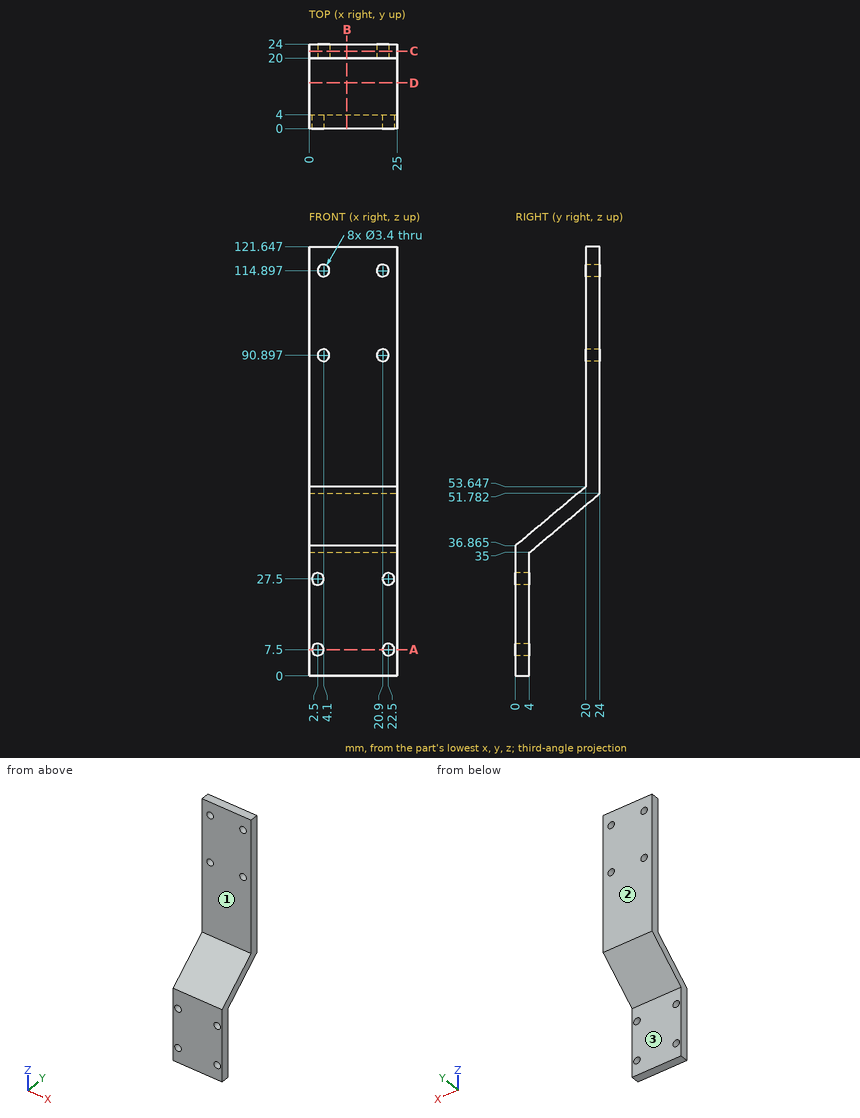
Verification items for this drawing (mm, ordinates from the low corner). A direction names the side the tool comes from. Give positions to 0.01 mm unless a question says otherwise; leave off trailing zeros. Loops run counter-clockwise (first coordinate to the right, second up) from the corner with the lowest first, then second, coordinate; pieces in that order, holes last. Notation, with made-up numbers: M -9,36.25 L 12,36.25 A16 cw 12,53.25 Z; hole C -25.5,18 d11. An arc over 180 degrees is marked long. Return JSON: item names as keys, results as strings. Group by question number.
1. Cross-section at B-B on x = 10.75. Record the boundary of the cut face in (y, z) (1 decimal), plus the area to 3 significant figures.
2. Cross-section at C-C on y = 22. Record the boundary of the cut face in (x, z), plus the area to 3 significant figures.
3. Cross-section at D-D on y = 13. Record the boundary of the cut face in (x, z), plus the area to 3 significant figures.
4. Tool access check on the marked faces 1, 2 and 3. Record the directions out of +Z, -Z, +X, -X, +Y, -Y that give a thin tool (end or side, any length) a straight path to the whole face; none if there is none.
5. Thickness scan on L1, parallel to X at y = 1.6, z = 7.5; L2, parallel to Z at x = 20.9, y = 22.6; L3, parallel to Z at x = 22.5, y = 2. Record the ranges inside material, lowest first.
6. Go/stop test with flat-tipped pins: pin 1 (10 mm diameter, centred on x = 20.5, y = 13.5, fed in from -Z); pin 2 (12 mm diameter, centred on x = 10.5, z = 80.5, fed in from -Y); pin 3 (4.5 mm diameter, centred on x = 4.1, z = 90.9, fed in from +Y); pin 4 (4 mm diameter, centred on x = 2.5, z = 7.5, fed in from +Y). Record where each tip stops, or that it passes through.
7. Cross-section at A-A on z = 7.5. Record the boundary of the cut face in (x, y).
Return value:
{
 "1": {"outline": "M 0,0 L 4,0 L 4,35 L 24,51.8 L 24,121.6 L 20,121.6 L 20,53.6 L 0,36.9 Z", "area": "524 mm^2"},
 "2": {"outline": "M 0,50.1 L 25,50.1 L 25,121.65 L 0,121.65 Z; hole C 4.1,90.9 d3.4; hole C 4.1,114.9 d3.4; hole C 20.9,90.9 d3.4; hole C 20.9,114.9 d3.4", "area": "1,750 mm^2"},
 "3": {"outline": "M 0,42.55 L 25,42.55 L 25,47.77 L 0,47.77 Z", "area": "131 mm^2"},
 "4": {"face 1": "+Z, +X, -X, -Y", "face 2": "+Z, -Z, +X, -X, +Y", "face 3": "-Z, +X, -X, +Y"},
 "5": {"L1": "0 to 0.8, 4.2 to 20.8, 24.2 to 25", "L2": "50.61 to 89.2, 92.6 to 113.2, 116.6 to 121.65", "L3": "0 to 5.8, 9.2 to 25.8, 29.2 to 38.54"},
 "6": {"pin 1": "z = 38.78", "pin 2": "y = 20", "pin 3": "y = 24", "pin 4": "y = 4"},
 "7": {"outline": "M 0,0 L 0.8,0 L 0.8,4 L 0,4 Z; M 4.2,0 L 20.8,0 L 20.8,4 L 4.2,4 Z; M 24.2,0 L 25,0 L 25,4 L 24.2,4 Z"}
}
